```python
from build123d import *

# Parameters (mm, degrees)
F0_W     = 110
F0_H     = 65
F0_R     = 1.5
F1_DEPTH = 1.6
F2_W     = 80
F2_H     = 58
F3_DEPTH = 5


with BuildPart() as f1:
    # F0 (on Front) → F1 (new body)
    with BuildSketch(Plane.XZ):
        with Locations((55, 32.5)):
            Rectangle(F0_W, F0_H)
        with Locations((4, 4)):
            Circle(F0_R, mode=Mode.SUBTRACT)
        with Locations((106, 4)):
            Circle(F0_R, mode=Mode.SUBTRACT)
        with Locations((4, 61)):
            Circle(F0_R, mode=Mode.SUBTRACT)
        with Locations((106, 61)):
            Circle(F0_R, mode=Mode.SUBTRACT)
    extrude(amount=F1_DEPTH)

    # F2 (on face) → F3 (join)
    with BuildSketch(Plane.XZ.offset(1.6)):
        with Locations((55, 32.5)):
            Rectangle(F2_W, F2_H)
    extrude(amount=F3_DEPTH)


solid = f1.part
```
Source: CAD feature listing. Evaluate the final solid. Frame: model axes, mm. A direction names the side the tool comes from. Give positions to 0.01 mm unless a question says otherwise; leave off trailing zeros. Order: outer loops, then holes, each group sorted by start corner. A loop starts at its lowest first (then second) coordinate and runs counter-clockwise, first axis right, second up.
(1) Section query C-C (y = -3). Return the cut outline in (x, z), plus the area to 3 significant figures.
(2) Access query for faces 1 (the face through (15, -4, 32)), 2 (the face through (54, -4, 61.5)), 3 (the face through (54, -6.6, 33)), 4 (the face through (95, -4, 32)), 5 (the face through (104.5, -0.79, 4.07)). Directions: +Z, -Z, +X, -X, +Y, -Y. A direction counts if a zero-diameter tool reaches every point of the face in a straight line with its end or side. Return the directions, or none.
(3) Section query A-A (x = 106). Return the cut outline in (y, z).
(4) Section query D-D (x = 67). Return the cut outline in (y, z).
(5) Material intervals for line 1 along Z through (x, y) = (106, -0.6); line 2 along Y through (x, z) = (7.5, 24.5); line 3 along Z through (x, y) = (68.5, -2), sorted ascending.
(6) Section query B-B (z = 14). Return the cut outline in (x, y), plus the area to 3 significant figures.
(7) Contact query for flat-ended pins moving along their axis: P1, Ø2.5, axis at x = 4, z = 61, coming from the -Y side; P2, Ø2.5, axis at x = 73, y = -3, coming from the -Z side; P3, Ø3.5, axis at x = 106, z = 61, coming from the -Y side; P4, Ø1.5, axis at y = -3, z = 34.5, coming from the -X side. Output: stop coordinate, or through.
(8) Pull-direction query (Z, two-part tool) for faces 6 (the face through (54, 0, 33)), 7 (the face through (3.805, -0.789, 62.487)), 8 (the face through (54, -4, 3.5)); classes: +Z half, -Z half, draft (parallel to the pull), parting line (faces both ways), or undercut.
Outcome:
1. outline: (15, 3.5) - (95, 3.5) - (95, 61.5) - (15, 61.5) - close
1. area: 4,640 mm2
2. face 1: +Z, -Z, -X, -Y
2. face 2: +Z, +X, -X, -Y
2. face 3: +Z, -Z, +X, -X, -Y
2. face 4: +Z, -Z, +X, -Y
2. face 5: +Y, -Y
3. outline: (-1.6, 0) - (0, 0) - (0, 2.5) - (-1.6, 2.5) - close; (-1.6, 5.5) - (0, 5.5) - (0, 59.5) - (-1.6, 59.5) - close; (-1.6, 62.5) - (0, 62.5) - (0, 65) - (-1.6, 65) - close
4. outline: (-6.6, 3.5) - (-1.6, 3.5) - (-1.6, 0) - (0, 0) - (0, 65) - (-1.6, 65) - (-1.6, 61.5) - (-6.6, 61.5) - close
5. line 1: z = 0 to 2.5, 5.5 to 59.5, 62.5 to 65
5. line 2: y = -1.6 to 0
5. line 3: z = 3.5 to 61.5
6. outline: (0, -1.6) - (15, -1.6) - (15, -6.6) - (95, -6.6) - (95, -1.6) - (110, -1.6) - (110, 0) - (0, 0) - close
6. area: 576 mm2
7. P1: passes through
7. P2: stops at z = 3.5
7. P3: stops at y = -1.6
7. P4: stops at x = 15
8. face 6: draft
8. face 7: undercut
8. face 8: -Z half
